The model under review builds one solid part; all positions refer to its coordinate system, in mm. A direction names the side the tool comes from. Coordinates: 2 decimals unless noted, no trailing zeros. Loops run counter-clockwise (first coordinate to the right, second up) from the corner with the lowest first, then second, coordinate; pieces in that order, holes last. Notation, with made-up numbers: M -25,16 L 7,16 A6 ccw 7,26 Z; hole C -33.5,11 d2. An arc over 180 degrees is marked long. Return JSON: item names as keys, results as strings.
```python
from build123d import *

# Parameters (mm, degrees)
CROQUIS1_R              = 2.3
SALIENTE_EXTRUIR1_DEPTH = 8


with BuildPart() as part:
    # Croquis1 → Saliente-Extruir1 (new body)
    with BuildSketch(Plane.XY):
        with BuildLine():
            Line((3.627068375, 1.5), (7.475, 1.5))
            Line((7.475, 1.5), (7.475, -1.5))
            Line((7.475, -1.5), (3.627068375, -1.5))
            ThreePointArc((3.627068375, -1.5), (0, -3.925), (-3.627068375, -1.5))
            Line((-3.627068375, -1.5), (-7.475, -1.5))
            Line((-7.475, -1.5), (-7.475, 1.5))
            Line((-7.475, 1.5), (-3.627068375, 1.5))
            ThreePointArc((-3.627068375, 1.5), (0, 3.925), (3.627068375, 1.5))
        make_face()
        Circle(CROQUIS1_R, mode=Mode.SUBTRACT)
    extrude(amount=-SALIENTE_EXTRUIR1_DEPTH)


solid = part.part
```
1. Add section A-A on z = -5. Give the boundary of the cut face in (x, y) (3 decimals).
Check values:
{"outline": "M -7.475,-1.5 L -3.627,-1.5 A3.925 ccw 3.627,-1.5 L 7.475,-1.5 L 7.475,1.5 L 3.627,1.5 A3.925 ccw -3.627,1.5 L -7.475,1.5 Z; hole C 0,0 d4.6"}
2. Add section B-B on x = 0. Give the boundary of the cut face in (y, z) (3 decimals).
Check values:
{"outline": "M -3.925,-8 L -2.3,-8 L -2.3,0 L -3.925,0 Z; M 2.3,-8 L 3.925,-8 L 3.925,0 L 2.3,0 Z"}
3. Machinability: for faces 1 (the face through (6, 1.5, -4)), 2 (the face through (6, -1.5, -4)), 3 (the face through (-6, -1.5, -4)), 4 (the face through (-6, 1.5, -4)), which of the approach directions +Z, -Z, +X, -X, +Y, -Y give a long, thin tool a straight path to every point of the face, cutting with its end or side? Answer none if there is none.
Check values:
{"face 1": "+Z, -Z, +X, +Y", "face 2": "+Z, -Z, +X, -Y", "face 3": "+Z, -Z, -X, -Y", "face 4": "+Z, -Z, -X, +Y"}
4. The part is to be moulded in two halves that separate along X. For faces 5 (the face through (2, -2, 0)), 6 (the face through (-1.825, -1.4, -3.944)), 7 (the face through (0.065, -3.924, -3.944)), 8 (the face through (-7.475, 0, -4)), say which applies: released by +X, released by -X, zero draft, split by the parting line, or undercut.
Check values:
{"face 5": "zero draft", "face 6": "undercut", "face 7": "split by the parting line", "face 8": "released by -X"}
5. To check wall thickness, follow line 1 (Y direction, x = 0, z = -4.5) (3 decimals); line 2 (Y direction, x = 1.5, z = -7); line 3 (X direction, y = 0.75, z = -4.25) (3 decimals). State the ranges of each line that lie inside material, in increasing order.
Check values:
{"line 1": "-3.925 to -2.3, 2.3 to 3.925", "line 2": "-3.63 to -1.74, 1.74 to 3.63", "line 3": "-7.475 to -2.174, 2.174 to 7.475"}
6. Insertion check: pin 1 Ø1.9 at (x, z) = (-5, -3) entering from -Y; pin 2 Ø1.2 at (x, z) = (5, -3.5) entering from +Y; pin 3 Ø4 at (x, z) = (-5, -4) entering from +Y. Each pin has a flat end and moves straight along its axis. Give the tip position at first contact, or say it passes through.
Check values:
{"pin 1": "y = -1.5", "pin 2": "y = 1.5", "pin 3": "y = 2.53"}
7. Add section D-D on x = 6.75. Give the boundary of the cut face in (y, z), plus the area to 3 significant figures.
Check values:
{"outline": "M -1.5,-8 L 1.5,-8 L 1.5,0 L -1.5,0 Z", "area": "24.0 mm²"}
8. Add section C-C on y = 0. Give the boundary of the cut face in (x, z) (3 decimals), plus the area to 3 significant figures.
Check values:
{"outline": "M -7.475,-8 L -2.3,-8 L -2.3,0 L -7.475,0 Z; M 2.3,-8 L 7.475,-8 L 7.475,0 L 2.3,0 Z", "area": "82.8 mm²"}
